```python
from build123d import *

# Parameters (mm, degrees)
EXTRUDE_1_DEPTH     = 12
SKETCH_2_R          = 1
CUT_EXTRUDE_1_DEPTH = 3


with BuildPart() as part:
    # 草图1 → 凸台-拉伸1 (new body)
    with BuildSketch(Plane.XY):
        Polygon((0, 25.75), (0, 17.95), (15, 17.95), (15, -17.95), (0, -17.95), (0, -25.75), (2, -25.75), (2, -19.75), (17, -19.75), (17, 19.75), (2, 19.75), (2, 25.75), align=None)
    extrude(amount=EXTRUDE_1_DEPTH)

    # 草图2 → 切除-拉伸1 (cut)
    with BuildSketch(Plane.ZY):
        with Locations((6, 23.531116708)):
            Circle(SKETCH_2_R)
        with Locations((6, -22.75)):
            Circle(SKETCH_2_R)
    extrude(amount=-CUT_EXTRUDE_1_DEPTH, mode=Mode.SUBTRACT)


solid = part.part
```
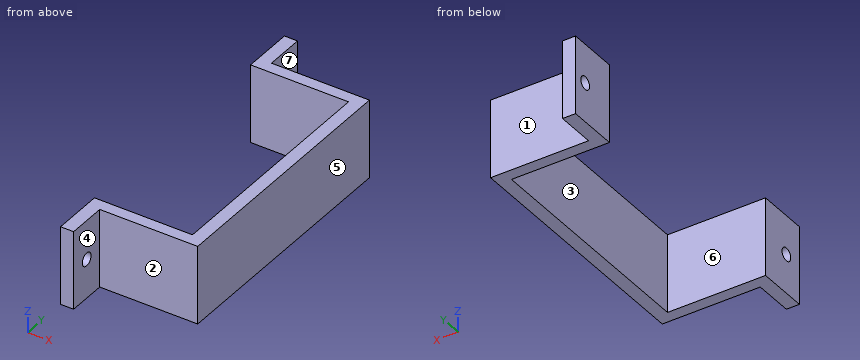
CAD build for the part. Positions are in the model's coordinates, mm. Face numbers are marked on the shaded views. A direction names the side the tool comes from. Round coordinates to 2 decimals unless told otherwise and drop trailing zeros. Loops run counter-clockwise (first coordinate to the right, second up) from the corner with the lowest first, then second, coordinate; pieces in that order, holes last. Notation, with made-up numbers: M 46,59 L 93,59 A22 ccw 93,83 Z; hole C 10.25,-11 d2. An arc over 180 degrees is marked long. Return JSON: item names as keys, results as strings. Group by question number.
(1) Saw through at D-D, the plane z = 9.5. List the corners of the cut face in (x, y), and give its area (3 significant figures).
(2) Wall check: probe 1 along Y at (x, z) = (0.5, 6); probe 2 along Y at (x, z) = (5.25, 6); probe 3 along X at (y, z) = (-9, 2.25). Give the ranges that are in metal, low to high. Write a range as [from, to].
(3) Saw through at A-A, the plane z = 6.5. List the corners of the cut face in (x, y).
(4) Drop flat-ended pins along their axis: P1, Ø1, axis at x = 10, z = 6, coming from the +Y side; P2, Ø2, axis at y = 17.5, z = 5.5, coming from the -X side; P3, Ø6.5, axis at y = -24, z = 3.5, coming from the +X side. Give the stop position or say it passes through.
(5) Saw through at C-C, the plane x = 12. List the corners of the cut face in (y, z).
(6) Saw through at B-B, the plane y = -22.75. List the corners of the cut face in (x, z).
(7) Tool access for the marked faces 5, 6 and 7: list every direction of +Z, -Z, +X, -X, +Y, -Y with a clear straight run to the whole face (end or side of a thin tool).
(8) Mould opens along Y. For the marked faces 1, 2, 3 and 4 say: +Y half, -Y half, draft (parallel to the pull), parting line (faces both ways), or undercut.
Answer list:
{
 "1": {"outline": "M 0,-25.75 L 2,-25.75 L 2,-19.75 L 17,-19.75 L 17,19.75 L 2,19.75 L 2,25.75 L 0,25.75 L 0,17.95 L 15,17.95 L 15,-17.95 L 0,-17.95 Z", "area": "157 mm2"},
 "2": {"probe 1": "[-25.75, -23.75], [-21.75, -17.95], [17.95, 22.53], [24.53, 25.75]", "probe 2": "[-19.75, -17.95], [17.95, 19.75]", "probe 3": "[15, 17]"},
 "3": {"outline": "M 0,-25.75 L 2,-25.75 L 2,-23.62 L 0,-23.62 Z; M 0,-21.88 L 2,-21.88 L 2,-19.75 L 17,-19.75 L 17,19.75 L 2,19.75 L 2,22.67 L 0,22.67 L 0,17.95 L 15,17.95 L 15,-17.95 L 0,-17.95 Z; M 0,24.4 L 2,24.4 L 2,25.75 L 0,25.75 Z"},
 "4": {"P1": "y = 19.75", "P2": "x = 0", "P3": "x = 2"},
 "5": {"outline": "M -19.75,0 L -17.95,0 L -17.95,12 L -19.75,12 Z; M 17.95,0 L 19.75,0 L 19.75,12 L 17.95,12 Z"},
 "6": {"outline": "M 0,0 L 2,0 L 2,5 L 0,5 Z; M 0,7 L 2,7 L 2,12 L 0,12 Z"},
 "7": {"face 5": "+Z, -Z, +X, +Y, -Y", "face 6": "+Z, -Z, -X", "face 7": "+Z, -Z, +X, +Y"},
 "8": {"face 1": "+Y half", "face 2": "-Y half", "face 3": "undercut", "face 4": "draft"}
}
